Input: part model. Units: mm. Frame: model coordinates. Give positions to 0.01 mm unless a question says otherwise; leave off trailing zeros. Loops run counter-clockwise (first coordinate to the right, second up) from the corner with the lowest first, then second, coordinate; pieces in that order, holes last. Notation, with made-up numbers: (21, 11) -> (43, 11) arc R15 ccw to (43, 31) -> close; hole circle Ø1 at (24, 19.5). An arc over 180 degrees is marked (long way). One line per question, with ' | ' between items.
from build123d import *

# Parameters (mm, degrees)
SKETCH_1_R      = 50
SKETCH_1_R_2    = 37.5
SKETCH_1_R_3    = 1.5
EXTRUDE_1_DEPTH = 1


with BuildPart() as part:
    # 草图1 → 凸台-拉伸1 (new body)
    with BuildSketch(Plane.XY):
        with Locations((-144.815895817, -92.623408185)):
            Circle(SKETCH_1_R)
        with Locations((-144.815895817, -92.623408185)):
            Circle(SKETCH_1_R_2, mode=Mode.SUBTRACT)
        with Locations((-190.167161981, -96.299364834)):
            Circle(SKETCH_1_R_3, mode=Mode.SUBTRACT)
        with Locations((-128.01669653, -134.908593573)):
            Circle(SKETCH_1_R_3, mode=Mode.SUBTRACT)
        with Locations(Location((-99.464629653, -88.947451536, 0), (0, 0, 180))):
            Circle(SKETCH_1_R_3, mode=Mode.SUBTRACT)
        with Locations(Location((-161.615095104, -50.338222797, 0), (0, 0, 180))):
            Circle(SKETCH_1_R_3, mode=Mode.SUBTRACT)
    extrude(amount=EXTRUDE_1_DEPTH)


solid = part.part
1. Ray query, line 1 along Y through (x, z) = (-138.5, 0.8); line 2 along Y through (x, z) = (-114, 0.85); line 3 along X through (y, z) = (-134, 0.85). Return the intervals inside material, ascending. Write a range as from..to.
Determined:
line 1: y = -142.22..-129.59, -55.66..-43.02 | line 2: y = -132..-113.99, -71.25..-53.25 | line 3: x = -172.89..-129.21, -126.82..-116.74
2. Pull-direction query (Y, two-part tool) for faces 1 (the flat face through (-138, -55, 0)), 2 (the cylindrical face through (-181.668, -58.831, 0.493)), 3 (the cylindrical face through (-163, -49.76, 0.49)); classes: pulls with the +Y half, pulls with the -Y half, needs draft (parallel to the pull), parting line crosses it, or undercut.
Determined:
face 1: needs draft | face 2: parting line crosses it | face 3: undercut
3. Section query C-C (z = 0.45). Output: boundary loops of the cut face in (x, y).
Determined:
outline: circle Ø100 at (-144.82, -92.62); hole circle Ø3 at (-190.17, -96.3); hole circle Ø75 at (-144.82, -92.62); hole circle Ø3 at (-161.62, -50.34); hole circle Ø3 at (-128.02, -134.91); hole circle Ø3 at (-99.46, -88.95)
4. Section query B-B (x = -181). Output: boundary loops of the cut face in (y, z), then the cut area to 3 significant figures.
Determined:
outline: (-127.13, 0) -> (-102.47, 0) -> (-102.47, 1) -> (-127.13, 1) -> close; (-82.78, 0) -> (-58.12, 0) -> (-58.12, 1) -> (-82.78, 1) -> close | area: 49.3 mm2
5. Section query A-A (y = -84). Output: boundary loops of the cut face in (x, z).
Determined:
outline: (-194.07, 0) -> (-181.31, 0) -> (-181.31, 1) -> (-194.07, 1) -> close; (-108.32, 0) -> (-95.57, 0) -> (-95.57, 1) -> (-108.32, 1) -> close
